Autodesk Inventor part; units mm, degrees
ref_plane "YZ Plane" through (0, 0, 0) normal (1, 0, 0) x (0, 1, 0)
ref_plane "XZ Plane" through (0, 0, 0) normal (0, 1, 0) x (-1, 0, 0)
ref_plane "XY Plane" through (0, 0, 0) normal (0, 0, 1) x (1, 0, 0)
sketch "Sketch1" plane through (0, 0, 0) normal (0, 0, 1) x (1, 0, 0)
  line L0 (0, 0) -> (50, 0)
  line L1 (50, 0) -> (50, 8.5)
  arc A0 (50, 8.5) -> (43.9926, 24) centre (27, 8.5) ccw
  line L2 (43.9926, 24) -> (0, 24)
  line L3 (0, 24) -> (0, 0)
  dimension "d0" = 50
  dimension "d1" = 24
  dimension "d2" = 8.5
  dimension "d3" = 23
extrude "Extrusion1" add sketch "Sketch1" along normal mid plane 39
sketch "Sketch2" plane through (0, 0, 0) normal (0, 0, 1) x (1, 0, 0)
  line L0 (0, 0) -> (0, 24)
  line L1 (0, 13.7) -> (26.2545, 13.7)
  arc A0 (26.2545, 5.7) -> (26.2545, 13.7) centre (26.2545, 9.7) ccw
  line L2 (26.2545, 5.7) -> (24, 5.7)
  line L3 (24, 5.7) -> (24, 0)
  line L4 (50, 0) -> (0, 0)
  line L5 (24, 0) -> (0, 0)
  line L6 (0, 0) -> (0, 13.7)
  line L7 (50, 8.5) -> (50, 0)
  dimension "d6" = 4
  dimension "d7" = 5.7
  dimension "d8" = 26
extrude "Extrusion2" cut sketch "Sketch2" along normal mid plane 31
sketch "Sketch3" plane through (0, 0, 0) normal (0, 0, 1) x (1, 0, 0)
  line L0 (14.5, 24.0258) -> (14.5, 18.2)
  line L1 (14.5, 18.2) -> (22, 18.2)
  line L2 (22, 18.2) -> (22, 0)
  line L3 (0, 13.7) -> (26.2545, 13.7)
  line L4 (22, 0) -> (45, 0)
  line L5 (50, 0) -> (0, 0)
  line L6 (50, 8.5) -> (50, 0)
  line L7 (50, 8.5) -> (50, 24.0258)
  line L8 (50, 24.0258) -> (14.5, 24.0258)
  line L9 (0, 24) -> (43.9926, 24)
  line L10 (45, 0) -> (48, 8.5)
  line L11 (48, 8.5) -> (50, 8.5)
  dimension "d11" = 2
  dimension "d12" = 5
  dimension "d13" = 8.5
  dimension "d14" = 4.5
  dimension "d15" = 35.5
  dimension "d16" = 28
extrude "Extrusion3" cut sketch "Sketch3" along normal mid plane 13 contours L8 L7 L11 L10 L4 L2 L1 L0
sketch "Sketch4" plane through (0, 24, -19.5) normal (0, 1, 0) x (1, 0, 0)
  line L0 (14.5, -26) -> (14.5, -13)
  line L1 (14.5, -13) -> (14.5, -26)
  arc A0 (14.5, -13) -> (14.5, -26) centre (14.5, -19.5) ccw
  point P0 (0, -19.5)
extrude "Extrusion4" cut sketch "Sketch4" against normal up to surface (5.8 mm away)
sketch "Sketch5" plane through (22, 18.2, 6.5) normal (0, 1, 0) x (1, 0, 0)
  arc A0 (-7.5, 13) -> (-7.5, 0) centre (-7.5, 6.5) ccw
  point P0 (-22, 6.5)
hole "Hole1" at (14.5, 18.2, 0) direction (0, -1, 0) diameter 5.2 end through all countersink diameter 9.5 countersink angle 90
chamfer "Chamfer1" distance 4 angle 45 3 edges at (21.9963, 24, 19.5) (0, 24, 0) (21.9963, 24, -19.5)
properties part number "Part015. Fixing Block" material "Steel, Carbon"
Part model, mm, in its own coordinate system. A direction names the side the tool comes from. Coordinates: 2 decimals unless noted, no trailing zeros. Order: outer loops, then holes, each group sorted by start corner. A loop starts at its lowest first (then second) coordinate and runs counter-clockwise, first axis right, second up. Notation, with made-up numbers: M -12.5,66 L -0.5,66 A15 cw -0.5,74 Z; hole C 17.5,73 d1. An arc over 180 degrees is marked long. One line per question, with ' | ' between items.
Q1. Two-plate mould, pull along X, no slides. Class faces 5 (the face through (50, 4, 0)), 6 (the face through (16.348, 16.184, -2.015)), 7 (the face through (46.48, 4.19, -0.09)), 8 (the face through (15, 7, -15.5)): +X half, -X half, draft (parallel to the pull), parting line (faces both ways), or undercut.
A:
face 5: +X half | face 6: undercut | face 7: -X half | face 8: draft
Q2. Pin check, flat tips, straight feed: P1, Ø4, axis at x = 12, z = 3, coming from the +Y side; P2, Ø5, axis at x = 37.5, z = 3, coming from the +Y side; P3, Ø1.3, axis at y = 16.5, z = 3, coming from the +X side; P4, Ø1.7, axis at y = 4, z = 10, coming from the -X side. Stop position of each tip, or through.
A:
P1: stops at y = 18.2 | P2: passes through | P3: stops at x = 22 | P4: stops at x = 24
Q3. Slice it at C-C (y = 9.7). Give the cut face in (x, z), and give its area (3 significant figures).
A:
outline: M 0,-19.5 L 49.97,-19.5 L 49.97,-6.5 L 30.25,-6.5 L 30.25,-15.5 L 0,-15.5 Z; M 0,15.5 L 30.25,15.5 L 30.25,6.5 L 49.97,6.5 L 49.97,19.5 L 0,19.5 Z | area: 755 mm^2
Q4. Slice it at D-D (z = 9). Give the cut face in (x, y).
A:
outline: M 0,13.7 L 26.25,13.7 A4 cw 26.25,5.7 L 24,5.7 L 24,0 L 50,0 L 50,8.5 A23 ccw 43.99,24 L 4,24 L 0,20 Z
Q5. Slice it at A-A (x = 36). Give the cut face in (y, z), and give its area (3 significant figures).
A:
outline: M 0,-19.5 L 20,-19.5 L 24,-15.5 L 24,-6.5 L 0,-6.5 Z; M 0,6.5 L 24,6.5 L 24,15.5 L 20,19.5 L 0,19.5 Z | area: 608 mm^2
Q6. Drill centre lines: line 1 (X direction, y = 14.5, z = 0); line 2 (Z direction, x = 16, y = 10.75); line 3 (Z direction, x = 14.5, y = 14.4). Where is each one in solid material? Low to high.
A:
line 1: x = 0 to 11.9, 17.1 to 22 | line 2: z = -19.5 to -15.5, 15.5 to 19.5 | line 3: z = -19.5 to -2.6, 2.6 to 19.5
Q7. Slice it at B-B (z = 0). Give the cut face in (x, y).
A:
outline: M 0,13.7 L 11.9,13.7 L 11.9,16.05 L 9.75,18.2 L 8,18.2 L 8,24 L 4,24 L 0,20 Z; M 17.1,13.7 L 22,13.7 L 22,18.2 L 19.25,18.2 L 17.1,16.05 Z; M 45,0 L 50,0 L 50,8.5 L 48,8.5 Z
Q8. 3-axis set-ups, long thin cutter, end or side, ignore diameter. For faces 1 (the face through (24, 3, 11)), 2 (the face through (8, 21, 0)), 3 (the face through (30, 0, -9)), 4 (the face through (25, 5.7, -11)): which of +Z, -Z, +X, -X, +Y, -Y reach the whole face in a straight line?
A:
face 1: -X, -Y | face 2: +X, +Y | face 3: +Z, -Z, +X, -X, -Y | face 4: -X
